Design review of the part shown in the three views and the two pictorial views. Dimensions are in mm from the part's minimum x, y and z. Coordinates: 2 decimals unless noted, no trailing zeros. Write each loop counter-clockwise with the first axis right and the second up, starting at its lowest first coordinate (ties: lowest second). Pieces come first, ordered by that corner, then holes. Notation, with made-up numbers: (24, 63.5) -> (66, 63.5) arc R14 ccw to (66, 86.5) -> close; hole circle Ø9 at (-10.75, 63.25). An arc over 180 degrees is marked (long way). Answer in a Markdown table with one row per item. Add a question column.
Item 1: Take a section at A-A, the plane z = 44.45. Write out the cut boundary in (x, y).
Item 2: Take a section at C-C, the plane y = 71. Write out the cut boundary in (x, z).
Item 3: Take a section at D-D, the plane z = 60.5. Write out the cut boundary in (x, y).
Item 4: To check wall thickness, follow line 1 (Z direction, x = 6, y = 3) (1 decimal); line 2 (Z direction, x = 2.5, y = 28.5); line 3 (Y direction, x = 2.5, z = 44.45). State the ranges of each line that lie inside material, in increasing order.
Item 5: Clearance check with flat-ended pins moving along their axes: P1, Ø1.9, axis at x = 2.5, y = 4.5, coming from the -Z side (3 decimals); P2, Ø1.8, axis at x = 2, y = 71, coming from the -Z side; P3, Ø1.9, axis at x = 4.5, z = 86.5, coming from the -Y side; P4, Ø5.5, axis at y = 28.575, z = 44.45, coming from the -X side. State where each tip first meets the part, or that it passes through.
Item 6: Take a section at B-B, the plane x = 5. Give the number of separate pieces and of enclosed holes in the cut face, and give its area (3 significant figures).
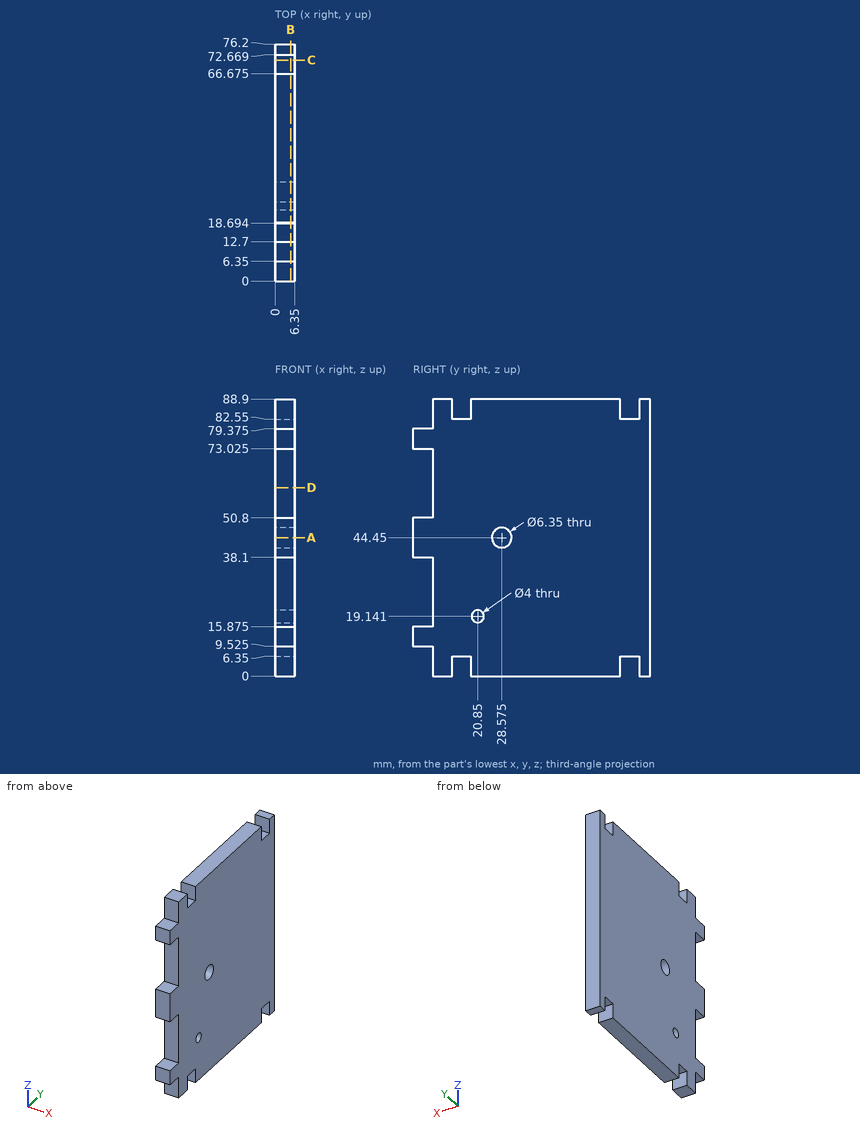
Answers:
| question | item | result |
|---|---|---|
| 1 | outline | (0, 0) -> (6.35, 0) -> (6.35, 25.4) -> (0, 25.4) -> close; (0, 31.75) -> (6.35, 31.75) -> (6.35, 76.2) -> (0, 76.2) -> close |
| 2 | outline | (0, 6.35) -> (6.35, 6.35) -> (6.35, 82.55) -> (0, 82.55) -> close |
| 3 | outline | (0, 6.35) -> (6.35, 6.35) -> (6.35, 76.2) -> (0, 76.2) -> close |
| 4 | line 1 | z = 9.5 to 15.9, 38.1 to 50.8, 73 to 79.4 |
| 4 | line 2 | z = 0 to 41.28, 47.62 to 88.9 |
| 4 | line 3 | y = 0 to 25.4, 31.75 to 76.2 |
| 5 | P1 | stops at z = 9.525 |
| 5 | P2 | stops at z = 6.35 |
| 5 | P3 | stops at y = 6.35 |
| 5 | P4 | passes through |
| 6 | separate pieces | 1 |
| 6 | enclosed holes | 2 |
| 6 | area | 6,170 mm^2 |
